Read the model definition and answer for the solid it produces. Units are mm, in the model's axes. A direction names the side the tool comes from. Give positions to 0.01 mm unless a question says otherwise; leave off trailing zeros. Order: outer loops, then holes, each group sorted by start corner. A loop starts at its lowest first (then second) coordinate and runs counter-clockwise, first axis right, second up. Notation, with made-up numbers: (24, 9) - (30, 9) arc R20 ccw to (30, 37) - close; hole circle Ø4 at (17.5, 31). An arc over 180 degrees is marked (long way). Use a Markdown table: item, result. Add a question column.
1. Consider L1, parallel to X at y = 7.5, z = -17.5; L2, parallel to Z at x = 0, y = 9.7; L3, parallel to X at y = 8.5, z = 0. Determine where each line is inside the solid, lowest interval first.
2. A cutting plane is placed at A-A on z = 0. Determine the outline of the cut face in (x, y), and give its area (3 significant figures).
3. A cutting plane is placed at B-B on x = 0. Determine the outline of the cut face in (y, z).
4. For a pull along X with two mould halves and no side action, classify faces 1 (the flat face through (-7.1, 10.5, -15.3)), 2 (the cylindrical face through (28.57, 6.8, -21)), 3 (the cylindrical face through (-23.265, 6.057, 17.728)) as released by +X, released by -X, zero draft, split by the parting line, or undercut.
5. Which of the six approach directions +Z, -Z, +X, -X, +Y, -Y give full straight-line access (tool end or side, diameter ignored) to faces 4 (the flat face through (19, 0, 1)), 5 (the flat face through (-25, 9.2, 18))?
6. A cutting plane is placed at C-C on y = 2. Determine the outline of the cut face in (x, z).
7. A cutting plane is placed at D-D on x = 20. Determine the outline of the cut face in (y, z), and give its area (3 significant figures).
8. Flat-ended cylindrical pins translate along their axes: P1, Ø20, axis at x = 0, z = 0, coming from the -Y side; P2, Ø2, axis at x = 17.5, z = 14.5, coming from the -Y side; P3, Ø1.8, axis at x = -25.5, z = 18, coming from the -Y side; P4, Ø4, axis at x = -0.5, z = -15.5, coming from the -Y side. Find the tip coordinate at first contact, or state that the pin passes through.
```python
from build123d import *

# Parameters (mm, degrees)
SKETCH1_R           = 21.25
SKETCH1_R_2         = 18.5
BOSS_EXTRUDE1_DEPTH = 8
SKETCH2_R           = 22.5
SKETCH2_R_2         = 16.5
BOSS_EXTRUDE2_DEPTH = 2.5
BOSS_EXTRUDE3_START = -7.5
SKETCH3_W           = 60
SKETCH3_H           = 45
SKETCH3_R           = 16.5
BOSS_EXTRUDE3_DEPTH = 7.5
FILLET2_R           = 5
SKETCH4_R           = 18.5
CUT_EXTRUDE1_DEPTH  = 4
SKETCH5_R           = 1.75
CUT_EXTRUDE2_DEPTH  = 6.2


with BuildPart() as part:
    # Sketch1 → Boss-Extrude1 (new body)
    with BuildSketch(Plane(origin=(0, 0, 0), x_dir=(1, 0, 0), z_dir=(0, 1, 0))):
        with Locations(Location((0, 0, 0), (0, 0, 270))):
            Circle(SKETCH1_R)
        with Locations(Location((0, 0, 0), (0, 0, 270))):
            Circle(SKETCH1_R_2, mode=Mode.SUBTRACT)
    extrude(amount=BOSS_EXTRUDE1_DEPTH)

    # Sketch2 → Boss-Extrude2 (add)
    with BuildSketch(Plane(origin=(0, 8, 0), x_dir=(1, 0, 0), z_dir=(0, 1, 0))):
        with Locations(Location((0, 0, 0), (0, 0, 270))):
            Circle(SKETCH2_R)
        with Locations(Location((0, 0, 0), (0, 0, 270))):
            Circle(SKETCH2_R_2, mode=Mode.SUBTRACT)
    extrude(amount=BOSS_EXTRUDE2_DEPTH)

    # Sketch3 → Boss-Extrude3 (add)
    with BuildSketch(Plane(origin=(0, 10.5, 0), x_dir=(1, 0, 0), z_dir=(0, 1, 0)).offset(BOSS_EXTRUDE3_START)):
        Rectangle(SKETCH3_W, SKETCH3_H)
        with Locations(Location((0, 0, 0), (0, 0, 270))):
            Circle(SKETCH3_R, mode=Mode.SUBTRACT)
    extrude(amount=BOSS_EXTRUDE3_DEPTH)

    # Fillet2
    fillet2_edges = [part.edges().sort_by_distance(p)[0] for p in [
        (30, 6.75, -22.5),
        (30, 6.75, 22.5),
        (-30, 6.75, 22.5),
        (-30, 6.75, -22.5),
    ]]
    fillet(fillet2_edges, radius=FILLET2_R)

    # Sketch4 → Cut-Extrude1 (cut)
    with BuildSketch(Plane(origin=(0, 3, 0), x_dir=(-1, 0, 0), z_dir=(0, -1, 0))):
        with Locations(Location((0, 0, 0), (0, 0, 90))):
            Circle(SKETCH4_R)
    extrude(amount=-CUT_EXTRUDE1_DEPTH, mode=Mode.SUBTRACT)

    # Sketch5 → Cut-Extrude2 (cut)
    with BuildSketch(Plane(origin=(0, 3, 0), x_dir=(-1, 0, 0), z_dir=(0, -1, 0))):
        with Locations(Location((25, -17.5, 0), (0, 0, 90))):
            Circle(SKETCH5_R)
        with Locations(Location((-25, -17.5, 0), (0, 0, 90))):
            Circle(SKETCH5_R)
        with Locations(Location((-25, 17.5, 0), (0, 0, 90))):
            Circle(SKETCH5_R)
        with Locations(Location((25, 17.5, 0), (0, 0, 90))):
            Circle(SKETCH5_R)
    extrude(amount=-CUT_EXTRUDE2_DEPTH, mode=Mode.SUBTRACT)


solid = part.part
```
Output values:
| question | item | result |
|---|---|---|
| 1 | L1 | -30 to -26.75, -23.25 to 23.25, 26.75 to 30 |
| 1 | L2 | -22.5 to -16.5, 16.5 to 22.5 |
| 1 | L3 | -30 to -16.5, 16.5 to 30 |
| 2 | outline | (-30, 3) - (-21.25, 3) - (-21.25, 0) - (-18.5, 0) - (-18.5, 7) - (-16.5, 7) - (-16.5, 10.5) - (-30, 10.5) - close; (16.5, 7) - (18.5, 7) - (18.5, 0) - (21.25, 0) - (21.25, 3) - (30, 3) - (30, 10.5) - (16.5, 10.5) - close |
| 2 | area | 203 mm² |
| 3 | outline | (0, -21.25) - (3, -21.25) - (3, -22.5) - (10.5, -22.5) - (10.5, -16.5) - (7, -16.5) - (7, -18.5) - (0, -18.5) - close; (0, 18.5) - (7, 18.5) - (7, 16.5) - (10.5, 16.5) - (10.5, 22.5) - (3, 22.5) - (3, 21.25) - (0, 21.25) - close |
| 4 | face 1 | zero draft |
| 4 | face 2 | released by +X |
| 4 | face 3 | undercut |
| 5 | face 4 | +Z, -Z, +X, -X, -Y |
| 5 | face 5 | -Y |
| 6 | outline | circle Ø42.5 at (0, 0); hole circle Ø37 at (0, 0) |
| 7 | outline | (0, -7.18) - (3, -7.18) - (3, -22.5) - (10.5, -22.5) - (10.5, 22.5) - (3, 22.5) - (3, 7.18) - (0, 7.18) - close |
| 7 | area | 381 mm² |
| 8 | P1 | through |
| 8 | P2 | y = 3 |
| 8 | P3 | y = 9.2 |
| 8 | P4 | y = 7 |
